from build123d import *

# Parameters (mm, degrees)
SKETCH1_R           = 1.55
BOSS_EXTRUDE1_DEPTH = 3


with BuildPart() as part:
    # Sketch1 → Boss-Extrude1 (new body)
    with BuildSketch(Plane.XY):
        with BuildLine():
            Line((-5.95, -2.354308425), (-3.45, -2.354308425))
            Line((-3.45, -2.354308425), (3.45, -2.354308425))
            Line((3.45, -2.354308425), (5.95, -2.354308425))
            Line((5.95, -2.354308425), (5.95, -2.154308425))
            ThreePointArc((5.95, -2.154308425), (4.323654403, -1.480654022), (3.65, 0.145691575))
            Line((3.65, 0.145691575), (3.65, 3))
            Line((3.65, 3), (3.65, 7))
            ThreePointArc((3.65, 7), (3.18137085, 8.13137085), (2.05, 8.6))
            Line((2.05, 8.6), (-2.05, 8.6))
            ThreePointArc((-2.05, 8.6), (-3.18137085, 8.13137085), (-3.65, 7))
            Line((-3.65, 7), (-3.65, 3))
            Line((-3.65, 3), (-3.65, 0.145691575))
            ThreePointArc((-3.65, 0.145691575), (-4.323654403, -1.480654022), (-5.95, -2.154308425))
            Line((-5.95, -2.154308425), (-5.95, -2.354308425))
        make_face()
        with Locations((0, 5)):
            Circle(SKETCH1_R, mode=Mode.SUBTRACT)
    extrude(amount=BOSS_EXTRUDE1_DEPTH)


solid = part.part
Model file for the job. Use its own axes, mm. A direction names the side the tool comes from. Give positions to 0.01 mm unless a question says otherwise; leave off trailing zeros. Loops run counter-clockwise (first coordinate to the right, second up) from the corner with the lowest first, then second, coordinate; pieces in that order, holes last. Notation, with made-up numbers: (57, 72) - (78, 72) arc R18 cw to (78, 89) - close; hole circle Ø7 at (-34.75, 55.25). An arc over 180 degrees is marked (long way). Use one line per item in the form item = value.
(1) Cut at D-D (y = 0.75). Give the cut face in (x, z), then the cut area to 3 significant figures.
Determined:
outline = (-3.65, 0) - (3.65, 0) - (3.65, 3) - (-3.65, 3) - close
area = 21.9 mm^2
(2) Cut at B-B (z = 0.7). Give the cut face in (x, y).
Determined:
outline = (-5.95, -2.35) - (5.95, -2.35) - (5.95, -2.15) arc R2.3 cw to (3.65, 0.15) - (3.65, 7) arc R1.6 ccw to (2.05, 8.6) - (-2.05, 8.6) arc R1.6 ccw to (-3.65, 7) - (-3.65, 0.15) arc R2.3 cw to (-5.95, -2.15) - close; hole circle Ø3.1 at (0, 5)
(3) Drop flat-ended pins along their axis: P1, Ø1.5, axis at y = 3, z = 2, coming from the -X side; P2, Ø3, axis at x = 0, y = 5, coming from the +Z side; P3, Ø1, axis at y = 0.5, z = 1.5, coming from the +X side; P4, Ø1, axis at x = 1.5, y = 3, coming from the -Z side. Give the stop position or say it passes through.
Determined:
P1 = -3.65
P2 = through
P3 = 3.65
P4 = 0
(4) Cut at C-C (y = 5). Give the cut face in (x, z), then the cut area to 3 significant figures.
Determined:
outline = (-3.65, 0) - (-1.55, 0) - (-1.55, 3) - (-3.65, 3) - close; (1.55, 0) - (3.65, 0) - (3.65, 3) - (1.55, 3) - close
area = 12.6 mm^2
(5) 3-axis set-ups, long thin cutter, end or side, ignore diameter. For faces 4 (the face through (3.65, 4, 1)), 5 (the face through (0, 3, 0)), 6 (the face through (-3.65, 4, 1)): which of +Z, -Z, +X, -X, +Y, -Y reach the whole face in a straight line?
Determined:
face_4 = +Z, -Z, +X, +Y
face_5 = -Z, +X, -X, +Y, -Y
face_6 = +Z, -Z, -X, +Y
(6) Pull direction Y, two halves, no side cores. Call faces 1 (the face through (0, 8.6, 1)), 2 (the face through (0.715, 3.625, 1.479)), 3 (the face through (0, 3, 3)): pulls with the +Y half, pulls with the -Y half, needs draft (parallel to the pull), parting line crosses it, or undercut.
Determined:
face_1 = pulls with the +Y half
face_2 = undercut
face_3 = needs draft
(7) Drill centre lines: L1, parallel to Y at x = 0, z = 1.7; L2, parallel to X at y = 2, z = 2.05; L3, parallel to X at y = -0.5, z = 1.95. Where is each one in solid material? Low to high.
Determined:
L1 = -2.35 to 3.45, 6.55 to 8.6
L2 = -3.65 to 3.65
L3 = -3.74 to 3.74
(8) Cut at A-A (x = 0). Give the cut face in (y, z), then the cut area to 3 significant figures.
Determined:
outline = (-2.35, 0) - (3.45, 0) - (3.45, 3) - (-2.35, 3) - close; (6.55, 0) - (8.6, 0) - (8.6, 3) - (6.55, 3) - close
area = 23.6 mm^2
